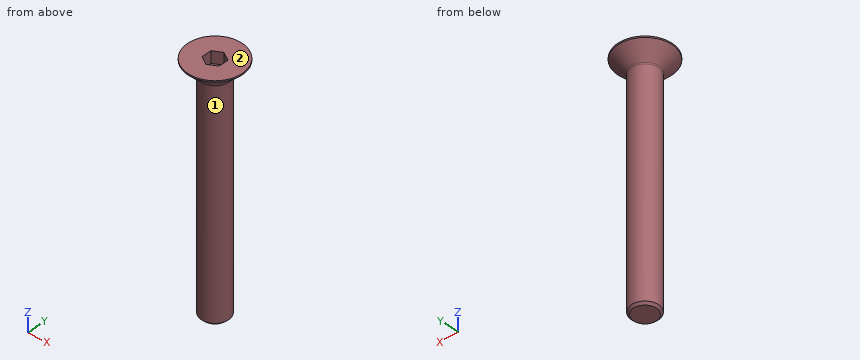
Autodesk Inventor part; units mm, degrees
ref_plane "MSC_PF1" through (0, 0, 0) normal (1, 0, 0) x (0, 1, 0)
ref_plane "MSC_PT1" through (0, 0, 0) normal (0, 0, -1) x (-1, 0, 0)
ref_plane "YZ Plane" through (0, 0, 0) normal (1, 0, 0) x (0, 1, 0)
sketch "Sketch1" plane through (0, 0, 0) normal (0, 1, 0) x (-1, 0, 0)
  point P0 (0, 0)
sketch "Sketch2" plane through (0, 0, 0) normal (0, 1, 0) x (-1, 0, 0)
  line L0 (-4, -70) -> (0, -70)
  line L1 (-4, -4.4) -> (-4, -70)
  line L2 (-8, -0.4) -> (-4, -4.4)
  line L3 (-8, 0) -> (-8, -0.4)
  line L4 (0, 0) -> (-8, 0)
  line L5 (0, -70) -> (0, 0)
  line L6 (0, -70) -> (0, 0)
  line L7 (0, -84) -> (0, 14)
  line L8 (1.6, 0) -> (-9.6, 0)
  dimension "d3" = 8
  dimension "d5" = 4
  dimension "d7" = 70
  dimension "ParC" = 0.4
  dimension "d22" = 0
  dimension "d23" = 0
  dimension "d43" = 45
revolve "Revolution1" add sketch "Sketch2" angle 360 about axis through (0, 0, -70) along (0, 0, -1)
sketch "Sketch3" plane through (0, 0, 0) normal (0, 0, 1) x (1, 0, 0)
  line L0 (-2.5, 1.4434) -> (-2.5, -1.4434)
  line L1 (0, 2.8868) -> (-2.5, 1.4434)
  line L2 (2.5, 1.4434) -> (0, 2.8868)
  line L3 (2.5, -1.4434) -> (2.5, 1.4434)
  line L4 (0, -2.8868) -> (2.5, -1.4434)
  line L5 (-2.5, -1.4434) -> (0, -2.8868)
  circle A0 centre (0, 0) radius 2.5 construction
  circle A1 centre (0, 0) radius 4 construction
  dimension "d11" = 5
  dimension "d13" = 120
  dimension "d15" = 120
extrude "Extrusion1" cut sketch "Sketch3" against normal blind 3.5
fillet "Fillet1" radius 0.5 1 edges at (-4, 0, -4.4)
chamfer "Chamfer1" distance 0.625 angle 45 1 edges at (-4, 0, -70) measured on face at (-0.9596, 3.8832, -48.2024)
thread "Thread1"
ref_plane "MSC_PF1" through (0, 0, 0) normal (1, 0, 0) x (0, 1, 0)
ref_plane "MSC_PT1" through (0, 0, 0) normal (0, 0, -1) x (-1, 0, 0)
equation "\"d3\" = 0.5 * dk"
equation "\"d5\" = 0.5 * NND"
equation "\"d43\" = 0.5 * ang"
equation "\"d18\" = r"
equation "\"d19\" = 0.5 * PTC"
equation "\"d39\" = 0.5 * PTC"
equation "\"d11\" = ParS"
equation "\"d16\" = ParT"
equation "\"NND\" = 8"
equation "\"PTC\" = 1.25"
equation "\"dk\" = 16"
equation "\"ParK\" = 4.4"
equation "\"ParS\" = 5"
equation "\"ParT\" = 3.5"
equation "\"r\" = 0.5"
equation "\"ang\" = 90deg"
equation "\"THREADDIA\" = NND"
properties part number "DIN 7991 - M8x60" material "Steel, Mild"
Input: part model. Units: mm. Frame: model coordinates. Face numbers are marked on the shaded views. A direction names the side the tool comes from. Give positions to 0.01 mm unless a question says otherwise; leave off trailing zeros. Order: outer loops, then holes, each group sorted by start corner. A loop starts at its lowest first (then second) coordinate and runs counter-clockwise, first axis right, second up. Notation, with made-up numbers: M -22.5,21 L 3.5,21 A25 ccw 3.5,46 Z; hole C 40.5,-6 d11. An arc over 180 degrees is marked long. One line per question, with ' | ' between items.
1) Access query for the marked faces 1 and 2. Directions: +Z, -Z, +X, -X, +Y, -Y. A direction counts if a zero-diameter tool reaches every point of the face in a straight line with its end or side. Return the directions, or none.
Filled in:
face 1: -Z | face 2: +Z, +X, -X, +Y, -Y
2) Ray query, L1, parallel to Z at x = 0.5, y = 0.25; L2, parallel to Z at x = -1.5, y = 3.25; L3, parallel to Y at x = 0, z = -32.5. Return the intervals inside material, ascending.
Filled in:
L1: z = -70 to -3.5 | L2: z = -69.8 to 0 | L3: y = -4 to 4
3) Contact query for flat-ended pins moving along their axis: P1, Ø1.4, axis at y = -0.5, z = -1.5, coming from the +X side; P2, Ø6, axis at x = 5.5, z = -20, coming from the +Y side; P3, Ø3, axis at y = 0, z = -2, coming from the -X side. Output: stop coordinate, or through.
Filled in:
P1: stops at x = 7.58 | P2: stops at y = 3.12 | P3: stops at x = -7.9
4) Section A-A on z = -18.5. Output: boundary loops of the cut face in (x, y).
Filled in:
outline: C 0,0 d8
